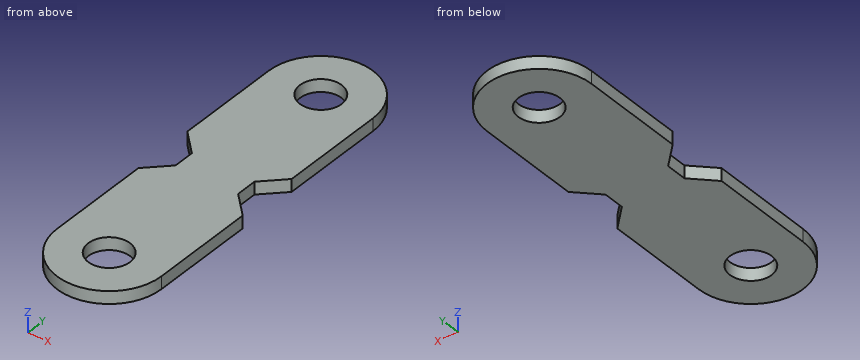
```python
from build123d import *

# Parameters (mm, degrees)
SKETCH_R     = 0.5
PAD_DEPTH    = 0.3
CHAMFER_SIZE = 0.499


with BuildPart() as part:
    # Sketch → Pad (new body)
    with BuildSketch(Plane.XY):
        with BuildLine():
            Line((-0.75, 0), (-0.75, -1.5))
            Line((-0.75, -1.5), (-1.25, -1.5))
            Line((-1.25, -1.5), (-1.25, -4))
            ThreePointArc((-1.25, -4), (0, -5.25), (1.25, -4))
            Line((1.25, -1.5), (1.25, -4))
            Line((0.75, -1.5), (1.25, -1.5))
            Line((0.75, 0), (0.75, -1.5))
            Line((0.75, 0), (1.25, 0))
            Line((1.25, 0), (1.25, 2.5))
            ThreePointArc((1.25, 2.5), (0, 3.75), (-1.25, 2.5))
            Line((-1.25, 0), (-1.25, 2.5))
            Line((-0.75, 0), (-1.25, 0))
        make_face()
        with Locations((0, -4)):
            Circle(SKETCH_R, mode=Mode.SUBTRACT)
        with Locations((0, 2.5)):
            Circle(SKETCH_R, mode=Mode.SUBTRACT)
    extrude(amount=PAD_DEPTH)

    # Chamfer
    chamfer_edges = [part.edges().sort_by_distance(p)[0] for p in [
        (-0.75, 0, 0.15),
        (-0.75, -1.5, 0.15),
        (0.75, 0, 0.15),
        (0.75, -1.5, 0.15),
    ]]
    chamfer(chamfer_edges, length=CHAMFER_SIZE)


solid = part.part
```
Can you work these out from the model? Positions are in its coordinate system, mm. Give positions to 0.01 mm unless a question says otherwise; leave off trailing zeros. Loops run counter-clockwise (first coordinate to the right, second up) from the corner with the lowest first, then second, coordinate; pieces in that order, holes last. Notation, with made-up numbers: M -8,54.25 L 24,54.25 A34 ccw 24,85.25 Z; hole C 74.25,46 d1. An arc over 180 degrees is marked long. Answer in a Markdown table with one row per item.
1. Suppose I cut it at D-D on x = -0.6. Write out the boundary of the cut face in (y, z), plus the area to 3 significant figures.
Taken from the geometry:
| item | result |
|---|---|
| outline | M -5.1,0 L 3.6,0 L 3.6,0.3 L -5.1,0.3 Z |
| area | 2.61 mm² |
2. Suppose I cut it at C-C on x = 0.65. Write out the boundary of the cut face in (y, z), plus the area to 3 significant figures.
Taken from the geometry:
| item | result |
|---|---|
| outline | M -5.07,0 L 3.57,0 L 3.57,0.3 L -5.07,0.3 Z |
| area | 2.59 mm² |
3. Suppose I cut it at A-A on x = 0. Write out the boundary of the cut face in (y, z).
Taken from the geometry:
| item | result |
|---|---|
| outline | M -5.25,0 L -4.5,0 L -4.5,0.3 L -5.25,0.3 Z; M -3.5,0 L 2,0 L 2,0.3 L -3.5,0.3 Z; M 3,0 L 3.75,0 L 3.75,0.3 L 3,0.3 Z |
4. Suppose I cut it at B-B on z = 0.2. Count the separate pieces of the cut face and the enclosed holes in it, plus the area to 3 significant figures.
Taken from the geometry:
| item | result |
|---|---|
| separate pieces | 1 |
| enclosed holes | 2 |
| area | 18.6 mm² |
5. If I drill on line 1 along Y through (x, z) = (0, 0.1); line 2 along X through (y, z) = (-3.75, 0.1); line 3 along Y through (x, z) = (0.85, 0.05), over which ranges is the centre line in solid material (lowest first)?
Taken from the geometry:
| item | result |
|---|---|
| line 1 | y = -5.25 to -4.5, -3.5 to 2, 3 to 3.75 |
| line 2 | x = -1.25 to -0.43, 0.43 to 1.25 |
| line 3 | y = -4.92 to -1.1, -0.4 to 3.42 |
